```python
from build123d import *

# Parameters (mm, degrees)
SKETCH1_W                    = 6.5
SKETCH1_H                    = 19
BOSS_BODY_DEPTH              = 3
SKETCH2_R                    = 0.65
CUT_SCREW_HOLES_DEPTH        = 4
SKETCH4_R                    = 1.25
CUT_SCREW_HEAD_POCKETS_DEPTH = 1.5


with BuildPart() as part:
    # Sketch1 → Boss-Body (new body)
    with BuildSketch(Plane(origin=(0, 0, 0), x_dir=(1, 0, 0), z_dir=(0, 1, 0))):
        Rectangle(SKETCH1_W, SKETCH1_H)
    extrude(amount=-BOSS_BODY_DEPTH)

    # Sketch2 → Cut-Screw Holes (cut, through all)
    with BuildSketch(Plane(origin=(0, 0, 0), x_dir=(1, 0, 0), z_dir=(0, 1, 0))):
        with Locations((0, -7.6)):
            Circle(SKETCH2_R)
        with Locations((0, 0.4)):
            Circle(SKETCH2_R)
        with Locations((0, 8.4)):
            Circle(SKETCH2_R)
        with Locations((0, 4.4)):
            Circle(SKETCH2_R)
        with Locations((0, -3.6)):
            Circle(SKETCH2_R)
    extrude(amount=-CUT_SCREW_HOLES_DEPTH, mode=Mode.SUBTRACT)

    # Sketch4 → Cut-Screw Head Pockets (cut)
    with BuildSketch(Plane(origin=(0, 0, 0), x_dir=(1, 0, 0), z_dir=(0, 1, 0))):
        with Locations((0, 4.4)):
            Circle(SKETCH4_R)
        with Locations((0, -3.6)):
            Circle(SKETCH4_R)
    extrude(amount=-CUT_SCREW_HEAD_POCKETS_DEPTH, mode=Mode.SUBTRACT)


solid = part.part
```
CAD build for the part. Positions are in the model's coordinates, mm. A direction names the side the tool comes from. Round coordinates to 2 decimals unless told otherwise and drop trailing zeros. Loops run counter-clockwise (first coordinate to the right, second up) from the corner with the lowest first, then second, coordinate; pieces in that order, holes last. Notation, with made-up numbers: (19.25, 57.5) - (34.25, 57.5) arc R22 ccw to (34.25, 77.5) - close; hole circle Ø8 at (64.5, 81.5). An arc over 180 degrees is marked (long way). Return JSON: item names as keys, results as strings. Group by question number.
Q1. Drill centre lines: line 1 along Z through (x, y) = (0, -2.55); line 2 along Z through (x, y) = (0, -1); line 3 along X through (y, z) = (-1.9, -0.4). Where is each one in solid material? Low to high. Write a range as [from, to].
Q2. Band-saw the part on C-C on x = 0. Give the number of separate pieces and of enclosed holes in the cut face, plus the area to 3 significant figures.
Q3. Flat gauge pins, fed straight in: pin 1 Ø0.8 at (x, z) = (0, 7.6) entering from +Y; pin 2 Ø2 at (x, z) = (0, -4.4) entering from +Y. Where does each tip first touch, or does it go through?
Q4. Band-saw the part on A-A on y = -0.4. Give the cut face in (x, z), plus the area to 3 significant figures.
Q5. Tool access for faces 5 (the face through (1, -1.5, 4)), 6 (the face through (0.35, -1.48, -8.95)): list every direction of +Z, -Z, +X, -X, +Y, -Y with a clear straight run to the whole face (end or side of a thin tool).
Q6. Band-saw the part on D-D on z = -0.4. Give the cut face in (x, y).
Q7. Band-saw the part on B-B on z = -4.4. Give the cut face in (x, y).
Q8. Two-plate mould, pull along Z, no slides. Class faces 1 (the face through (-3.25, -1, 0)), 2 (the face through (0, -1, 9.5)), 3 (the face through (-0.141, -1.479, 0.235)), 4 (the face through (0, -1, -9.5)): +Z half, -Z half, draft (parallel to the pull), parting line (faces both ways), or undercut.
Solutions:
{
 "1": {"line 1": "z = [-9.5, -9.05], [-7.75, -5.05], [-3.75, -1.05], [0.25, 2.95], [4.25, 6.95], [8.25, 9.5]", "line 2": "z = [-9.5, -9.05], [-7.75, -5.65], [-3.15, -1.05], [0.25, 2.35], [4.85, 6.95], [8.25, 9.5]", "line 3": "x = [-3.25, -0.65], [0.65, 3.25]"},
 "2": {"separate pieces": "6", "enclosed holes": "0", "area": "33.9 mm^2"},
 "3": {"pin 1": "passes through", "pin 2": "stops at y = -1.5"},
 "4": {"outline": "(-3.25, -9.5) - (3.25, -9.5) - (3.25, 9.5) - (-3.25, 9.5) - close; hole circle Ø2.5 at (0, -4.4); hole circle Ø2.5 at (0, 3.6); hole circle Ø1.3 at (0, -8.4); hole circle Ø1.3 at (0, -0.4); hole circle Ø1.3 at (0, 7.6)", "area": "110 mm^2"},
 "5": {"face 5": "+Y", "face 6": "+Y, -Y"},
 "6": {"outline": "(-3.25, -3) - (-0.65, -3) - (-0.65, 0) - (-3.25, 0) - close; (0.65, -3) - (3.25, -3) - (3.25, 0) - (0.65, 0) - close"},
 "7": {"outline": "(-3.25, -3) - (-0.65, -3) - (-0.65, -1.5) - (-1.25, -1.5) - (-1.25, 0) - (-3.25, 0) - close; (0.65, -3) - (3.25, -3) - (3.25, 0) - (1.25, 0) - (1.25, -1.5) - (0.65, -1.5) - close"},
 "8": {"face 1": "draft", "face 2": "+Z half", "face 3": "undercut", "face 4": "-Z half"}
}
